Geometry check sheet. Reference: the model listing, model coordinates, mm. Face numbers are marked on the shaded views. A direction names the side the tool comes from. Give positions to 0.01 mm unless a question says otherwise; leave off trailing zeros. Write each loop counter-clockwise with the first axis right and the second up, starting at its lowest first coordinate (ties: lowest second). Pieces come first, ordered by that corner, then holes. Notation, with made-up numbers: M -34,-12.5 L -15,-12.5 A30 ccw -15,9.5 Z; hole C -0.5,38 d8. An arc over 180 degrees is marked long. Write each question's results on one line, items separated by ' | '.
```python
from build123d import *

# Parameters (mm, degrees)
BOSS_EXTRUDE1_DEPTH     = 21
CUT_EXTRUDE1_DEPTH      = 306.614135799
CUT_EXTRUDE1_DEPTH_BACK = 306.614135799
SKETCH3_R               = 6


with BuildPart() as part:
    # Sketch1 → Boss-Extrude1 (new, symmetric)
    with BuildSketch(Plane(origin=(0, 0, 0), x_dir=(0, 0, -1), z_dir=(1, 0, 0))):
        Polygon((-120, 0), (-100, 0), (-100, -160), (100, -160), (100, 0), (120, 0), (120, -180), (-120, -180), align=None)
    extrude(amount=BOSS_EXTRUDE1_DEPTH, both=True)

    # Sketch2 → Revolve1 (revolve)
    with BuildSketch(Plane.XY, mode=Mode.PRIVATE) as revolve1_sk:
        Polygon((0, -180), (150, -180), (79.954646314, -220), (0, -220), align=None)
    revolve(revolve1_sk.sketch.rotate(Axis((0, 87.726376394, 0), (0, -1, 0)), 90), axis=Axis((0, 87.726376394, 0), (0, -1, 0)))

    # Sketch3 → Cut-Extrude1 (cut, two sides: drawn at the far end of the back side and taken through both)
    with BuildSketch(Plane.XY.offset(-CUT_EXTRUDE1_DEPTH_BACK)):
        Circle(SKETCH3_R)
    extrude(amount=CUT_EXTRUDE1_DEPTH + CUT_EXTRUDE1_DEPTH_BACK, mode=Mode.SUBTRACT)


solid = part.part
```
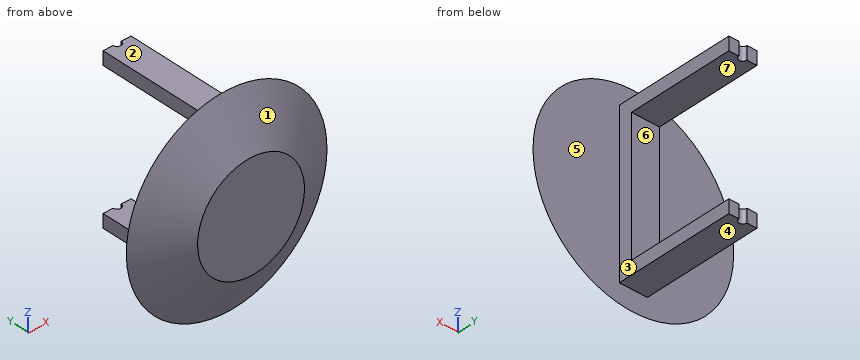
Q1. Section check A-A (y = -36.5). Enter the section's corners in (x, z), then the cut area to 3 significant figures.
Answer key:
outline: M -21,-120 L 21,-120 L 21,-100 L -21,-100 Z; M -21,100 L 21,100 L 21,120 L -21,120 Z | area: 1,680 mm2
Q2. Access from +Z, -Z, +X, -X, +Y, -Y to the whole of each face (thin tool, end or side, straight path). Record for the marked faces 1, 2 and 3.
Answer key:
face 1: -Y | face 2: +Z, +X, -X, +Y | face 3: +Z, -Z, +X, +Y
Q3. Section check D-D (y = -202). Enter the section's corners in (x, z).
Answer key:
outline: C 0,0 d222.95
Q4. Material ranges on probe 1 along Z at (x, y) = (13, -32); probe 2 along Y at (x, z) = (-58, -54.5); probe 3 along X at (y, z) = (-78, -113.5), recorded low to high. Write a range as [from, to].
Answer key:
probe 1: z = [-120, -100], [100, 120] | probe 2: y = [-220, -180] | probe 3: x = [-21, 21]
Q5. Release check for a two-part mould opening along Z. For the marked faces 4, 5, 6 and 7 record: released by +Z, released by -Z, zero draft, split by the parting line, or undercut.
Answer key:
face 4: released by -Z | face 5: zero draft | face 6: undercut | face 7: undercut
Q6. Depth check by flat-ended pin: P1, Ø21, axis at x = -6, y = -82.5, coming from the -Z side; P2, Ø1, axis at x = -91, z = -74, coming from the -Y side; P3, Ø1, axis at x = 13, z = -5, coming from the +Y side. Enter the tip coordinate at first touch or a pass-through.
Answer key:
P1: stops at z = -120 | P2: stops at y = -198.96 | P3: stops at y = -160
Q7. Section check B-B (x = 0). Enter the section's corners in (y, z), then the cut area to 3 significant figures.
Answer key:
outline: M -220,-79.95 L -180,-150 L -180,-120 L -6,-120 L -6,-100 L -160,-100 L -160,100 L -6,100 L -6,120 L -180,120 L -180,150 L -220,79.95 Z | area: 20,200 mm2
Q8. Section check C-C (z = 0). Enter the section's corners in (x, y), then the cut area to 3 significant figures.
Answer key:
outline: M -150,-180 L -79.95,-220 L 79.95,-220 L 150,-180 L 21,-180 L 21,-160 L -21,-160 L -21,-180 Z | area: 10,000 mm2
